Work out the finished part from the listing and answer in its coordinate system (mm). Face numbers are marked on the shaded views. A direction names the side the tool comes from. Round coordinates to 2 decimals unless told otherwise and drop trailing zeros. Write each loop counter-clockwise with the first axis right and the second up, starting at its lowest first coordinate (ties: lowest second). Pieces come first, ordered by that corner, then holes. Notation, with made-up numbers: (43.5, 56) -> (62.5, 56) arc R12 cw to (62.5, 68) -> close; hole circle Ø6 at (40.25, -17.5). An arc over 180 degrees is marked (long way). Answer as a JSON object with one key per item and string values. Group by question number.
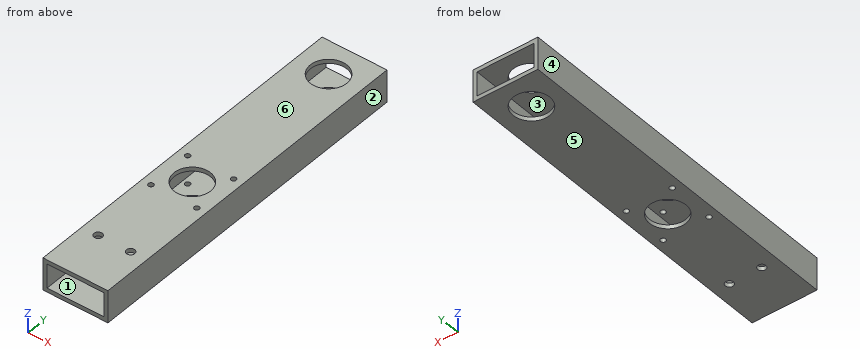
Autodesk Inventor part; units mm, degrees
ref_plane "YZ Plane" through (0, 0, 0) normal (1, 0, 0) x (0, 1, 0)
ref_plane "XZ Plane" through (0, 0, 0) normal (0, 1, 0) x (-1, 0, 0)
ref_plane "XY Plane" through (0, 0, 0) normal (0, 0, 1) x (1, 0, 0)
sketch "Sketch1" plane through (0, 0, 0) normal (0, 1, 0) x (-1, 0, 0)
  line L0 (25.4, 12.7) -> (-25.4, 12.7)
  line L1 (-25.4, 12.7) -> (-25.4, -12.7)
  line L2 (-25.4, -12.7) -> (25.4, -12.7)
  line L3 (25.4, -12.7) -> (25.4, 12.7)
  line L4 (25.4, 12.7) -> (-25.4, -12.7) construction
  line L5 (-25.4, 12.7) -> (25.4, -12.7) construction
  line L6 (22.225, 9.525) -> (-22.225, 9.525)
  line L7 (-22.225, 9.525) -> (-22.225, -9.525)
  line L8 (-22.225, -9.525) -> (22.225, -9.525)
  line L9 (22.225, -9.525) -> (22.225, 9.525)
  line L10 (22.225, 9.525) -> (-22.225, -9.525) construction
  line L11 (-22.225, 9.525) -> (22.225, -9.525) construction
  point P0 (0, 0)
  dimension "d0" = 50.8
  dimension "d1" = 25.4
  dimension "d2" = 44.45
  dimension "d3" = 19.05
extrude "Extrusion1" add sketch "Sketch1" along normal blind 273.05
sketch "Sketch2" plane through (-25.4, 0, 12.7) normal (0, 0, 1) x (1, 0, 0)
  line L0 (0, 0) -> (0, 273.05)
  line L1 (25.4, 0) -> (25.4, 38.1)
  line L2 (25.4, 0) -> (63.5, 0) construction
  line L3 (25.4, 38.1) -> (38.1, 38.1)
  line L4 (38.1, 38.1) -> (12.7, 38.1)
  circle A0 centre (12.7, 38.1) radius 3.175
  circle A1 centre (38.1, 38.1) radius 3.175
  dimension "d6" = 38.1
  dimension "d7" = 90
  dimension "d8" = 12.7
  dimension "d9" = 90
  dimension "d10" = 25.4
  dimension "d11" = 0
  dimension "d12" = 6.35
  dimension "d13" = 6.35
extrude "Extrusion2" cut sketch "Sketch2" against normal blind 203.2
sketch "Sketch3" plane through (-25.4, 0, 12.7) normal (0, 0, 1) x (1, 0, 0)
  line L0 (0, 273.05) -> (50.8, 273.05)
  line L1 (0, 0) -> (0, 273.05)
  line L2 (25.4, 273.05) -> (25.4, 247.65)
  line L3 (25.4, 273.05) -> (50.8, 273.05) construction
  circle A0 centre (25.4, 247.65) radius 14.2875
  point P0 (25.4, 0)
  dimension "d16" = 25.4
  dimension "d17" = 90
  dimension "d18" = 28.575
extrude "Extrusion3" cut sketch "Sketch3" against normal blind 25.4
sketch "Sketch4" plane through (-25.4, 0, 12.7) normal (0, 0, 1) x (1, 0, 0)
  line L0 (0, 0) -> (50.8, 0)
  line L1 (50.8, 0) -> (50.8, 76.2)
  line L2 (0, 76.2) -> (0, 0)
  line L3 (50.8, 76.2) -> (0, 76.2)
  line L4 (0, 76.2) -> (0, 127)
  line L5 (50.8, 127) -> (50.8, 76.2)
  circle A0 centre (25.4, 114.3) radius 14.2875
  line L6 (25.4, 114.3) -> (50.8, 114.3) construction
  circle A1 centre (7.4395, 132.2605) radius 2.032
  circle A2 centre (7.4395, 96.3395) radius 2.032
  circle A3 centre (43.3605, 96.3395) radius 2.032
  circle A4 centre (43.3605, 132.2605) radius 2.032
  point P0 (25.4, 0)
  dimension "d21" = 50.8
  dimension "d22" = 76.2
  dimension "d23" = 50.8
  dimension "d24" = 50.8
  dimension "d25" = 28.575
  dimension "d29" = 4.064
  dimension "d30" = 4.064
  dimension "d31" = 4.064
  dimension "d32" = 4.064
  dimension "d35" = 38.1
  dimension "d36" = 56.0605
  dimension "d37" = 56.0605
  dimension "d38" = 20.1395
  dimension "d39" = 20.1395
extrude "Extrusion4" cut sketch "Sketch4" against normal blind 25.4 contours A0 | A1 | A2 | A3 | A4
properties part number "ArmSupport"
1) A cutting plane is placed at A-A on z = -2.75. Determine the outline of the cut face in (x, y) (3 decimals).
2) A cutting plane is placed at B-B on y = 114.3. Determine the outline of the cut face in (x, z) (1 decimal), plus the area to 3 significant figures.
3) A cutting plane is placed at D-D on x = -1. Determine the outline of the cut face in (y, z) (3 decimals), plus the area to 3 significant figures.
4) A tool of negligible diameter and unlimited length cuts with its end or side. For the marked faces 1 and 2, from which of +Z, -Z, +X, -X, +Y, -Y can it reach the whole face along a straight path? Write none if from no direction.
5) Straight lines are drawn through the part: L1, parallel to Z at x = 15, y = 53 (3 decimals); L2, parallel to X at y = 172, z = 5.5 (3 decimals); L3, parallel to Y at x = 12.7, z = -11.85 (3 decimals). For each, find the intervals that lie inside material, in ascending order.
6) For a pull along Z with two mould halves and no side action, classify the marked faces 3, 4, 5 and 6 as released by +Z, released by -Z, zero draft, split by the parting line, or undercut.
7) A cutting plane is placed at C-C on y = 38.1. Determine the outline of the cut face in (x, z) (3 decimals), plus the area to 3 significant figures.
Established:
{
 "1": {"outline": "(-25.4, 0) -> (-22.225, 0) -> (-22.225, 273.05) -> (-25.4, 273.05) -> close; (22.225, 0) -> (25.4, 0) -> (25.4, 273.05) -> (22.225, 273.05) -> close"},
 "2": {"outline": "(-25.4, -12.7) -> (-14.3, -12.7) -> (-14.3, -9.5) -> (-22.2, -9.5) -> (-22.2, 9.5) -> (-14.3, 9.5) -> (-14.3, 12.7) -> (-25.4, 12.7) -> close; (14.3, -12.7) -> (25.4, -12.7) -> (25.4, 12.7) -> (14.3, 12.7) -> (14.3, 9.5) -> (22.2, 9.5) -> (22.2, -9.5) -> (14.3, -9.5) -> close", "area": "262 mm²"},
 "3": {"outline": "(0, -12.7) -> (100.048, -12.7) -> (100.048, -9.525) -> (0, -9.525) -> close; (0, 9.525) -> (100.048, 9.525) -> (100.048, 12.7) -> (0, 12.7) -> close; (128.552, -12.7) -> (233.398, -12.7) -> (233.398, -9.525) -> (128.552, -9.525) -> close; (128.552, 9.525) -> (233.398, 9.525) -> (233.398, 12.7) -> (128.552, 12.7) -> close; (261.902, -12.7) -> (273.05, -12.7) -> (273.05, -9.525) -> (261.902, -9.525) -> close; (261.902, 9.525) -> (273.05, 9.525) -> (273.05, 12.7) -> (261.902, 12.7) -> close", "area": "1,370 mm²"},
 "4": {"face 1": "+Y, -Y", "face 2": "+Z, -Z, +X, +Y, -Y"},
 "5": {"L1": "z = -12.7 to -9.525, 9.525 to 12.7", "L2": "x = -25.4 to -22.225, 22.225 to 25.4", "L3": "y = 0 to 34.925, 41.275 to 107.755, 120.845 to 241.105, 254.195 to 273.05"},
 "6": {"face 3": "undercut", "face 4": "zero draft", "face 5": "released by -Z", "face 6": "released by +Z"},
 "7": {"outline": "(-25.4, -12.7) -> (-15.875, -12.7) -> (-15.875, -9.525) -> (-22.225, -9.525) -> (-22.225, 9.525) -> (-15.875, 9.525) -> (-15.875, 12.7) -> (-25.4, 12.7) -> close; (-9.525, -12.7) -> (9.525, -12.7) -> (9.525, -9.525) -> (-9.525, -9.525) -> close; (-9.525, 9.525) -> (9.525, 9.525) -> (9.525, 12.7) -> (-9.525, 12.7) -> close; (15.875, -12.7) -> (25.4, -12.7) -> (25.4, 12.7) -> (15.875, 12.7) -> (15.875, 9.525) -> (22.225, 9.525) -> (22.225, -9.525) -> (15.875, -9.525) -> close", "area": "363 mm²"}
}
